For this review, take the finished solid that the model builds, in its own axes (mm). A direction names the side the tool comes from. Coordinates: 2 decimals unless noted, no trailing zeros. Write each loop counter-clockwise with the first axis right and the second up, starting at its lowest first coordinate (ties: lowest second). Pieces come first, ordered by that corner, then holes.
```python
from build123d import *

# Parameters (mm, degrees)
ESBO_O1_W                = 74
ESBO_O1_H                = 20
RESSALTO_EXTRUS_O1_DEPTH = 11
ESBO_O4_W                = 72
ESBO_O4_H                = 9.1
ESBO_O5_W                = 3
ESBO_O5_H                = 3
CORTE_EXTRUS_O2_DEPTH    = 2.5
CORTE_EXTRUS_O3_DEPTH    = 40.874804075
FILETE1_R                = 1
FILETE2_R                = 1
FILETE3_R                = 1
FILETE4_R                = 1
ESBO_O8_W                = 3.2
ESBO_O8_H                = 2
CORTE_EXTRUS_O5_DEPTH    = 44.474130264
FILETE5_R                = 0.5
FILETE6_R                = 0.5
FILETE7_R                = 0.5
FILETE8_R                = 0.5
FILETE5_OF_ESPELHAR3_R   = 0.5
FILETE6_OF_ESPELHAR3_R   = 0.5
FILETE7_OF_ESPELHAR3_R   = 0.5
FILETE8_OF_ESPELHAR3_R   = 0.5


with BuildPart() as part:
    # Esboço1 → Ressalto-extrusão1 (new body)
    with BuildSketch(Plane(origin=(0, 0, 0), x_dir=(1, 0, 0), z_dir=(0, 1, 0))):
        Rectangle(ESBO_O1_W, ESBO_O1_H)
    extrude(amount=RESSALTO_EXTRUS_O1_DEPTH)

    # Esboço4 → Corte-Revolução2 (revolve, cut)
    with BuildSketch(Plane(origin=(0, 11, 0), x_dir=(1, 0, 0), z_dir=(0, 1, 0))):
        with Locations((0, -4.55)):
            Rectangle(ESBO_O4_W, ESBO_O4_H)
    revolve(axis=Axis((-38.336087416, 11, 0), (1, 0, 0)), mode=Mode.SUBTRACT)

    # Esboço5 → Corte-extrusão2 (cut)
    with BuildSketch(Plane(origin=(-36, 0, 0), x_dir=(0, 0, -1), z_dir=(1, 0, 0))):
        with Locations((0, 8)):
            Rectangle(ESBO_O5_W, ESBO_O5_H)
    corte_extrus_o2 = extrude(amount=-CORTE_EXTRUS_O2_DEPTH, mode=Mode.SUBTRACT)

    # Espelhar1: Corte-extrusão2 across plane
    add(corte_extrus_o2.mirror(Plane(origin=(0, 0, 0), x_dir=(0, 0, 1), z_dir=(1, 0, 0))), mode=Mode.SUBTRACT)

    # Esboço6 → Corte-extrusão3 (cut, through all)
    with BuildSketch(Plane(origin=(0, 0, 0), x_dir=(1, 0, 0), z_dir=(0, 1, 0))):
        with BuildLine():
            Line((-36, 2), (-36, -2))
            ThreePointArc((-36, -2), (-34, 0), (-36, 2))
        make_face()
    corte_extrus_o3 = extrude(amount=CORTE_EXTRUS_O3_DEPTH, mode=Mode.SUBTRACT)

    # Filete1
    filete1_edges = [part.edges().sort_by_distance(p)[0] for p in [
        (37, 5.5, 10),
    ]]
    fillet(filete1_edges, radius=FILETE1_R)

    # Filete2
    filete2_edges = [part.edges().sort_by_distance(p)[0] for p in [
        (37, 5.5, -10),
    ]]
    fillet(filete2_edges, radius=FILETE2_R)

    # Filete3
    filete3_edges = [part.edges().sort_by_distance(p)[0] for p in [
        (-37, 5.5, 10),
    ]]
    fillet(filete3_edges, radius=FILETE3_R)

    # Filete4
    filete4_edges = [part.edges().sort_by_distance(p)[0] for p in [
        (-37, 5.5, -10),
    ]]
    fillet(filete4_edges, radius=FILETE4_R)

    # Espelhar2: Corte-extrusão3 across plane
    add(corte_extrus_o3.mirror(Plane(origin=(0, 0, 0), x_dir=(0, 0, 1), z_dir=(1, 0, 0))), mode=Mode.SUBTRACT)

    # Esboço8 → Corte-extrusão5 (cut, through all)
    with BuildSketch(Plane.XY.offset(10)):
        with Locations((-26.6, 2)):
            Rectangle(ESBO_O8_W, ESBO_O8_H)
    corte_extrus_o5 = extrude(amount=-CORTE_EXTRUS_O5_DEPTH, mode=Mode.SUBTRACT)

    # Filete5
    filete5_edges = [part.edges().sort_by_distance(p)[0] for p in [
        (-28.2, 2, 10),
    ]]
    fillet(filete5_edges, radius=FILETE5_R)

    # Filete6
    filete6_edges = [part.edges().sort_by_distance(p)[0] for p in [
        (-25, 2, 10),
    ]]
    fillet(filete6_edges, radius=FILETE6_R)

    # Filete7
    filete7_edges = [part.edges().sort_by_distance(p)[0] for p in [
        (-25, 2, -10),
    ]]
    fillet(filete7_edges, radius=FILETE7_R)

    # Filete8
    filete8_edges = [part.edges().sort_by_distance(p)[0] for p in [
        (-28.2, 2, -10),
    ]]
    fillet(filete8_edges, radius=FILETE8_R)

    # Espelhar3: Corte-extrusão5 across plane
    add(corte_extrus_o5.mirror(Plane(origin=(0, 0, 0), x_dir=(0, 0, 1), z_dir=(1, 0, 0))), mode=Mode.SUBTRACT)

    # Filete5 of Espelhar3
    filete5_of_espelhar3_edges = [part.edges().sort_by_distance(p)[0] for p in [
        (28.2, 2, 10),
    ]]
    fillet(filete5_of_espelhar3_edges, radius=FILETE5_OF_ESPELHAR3_R)

    # Filete6 of Espelhar3
    filete6_of_espelhar3_edges = [part.edges().sort_by_distance(p)[0] for p in [
        (25, 2, 10),
    ]]
    fillet(filete6_of_espelhar3_edges, radius=FILETE6_OF_ESPELHAR3_R)

    # Filete7 of Espelhar3
    filete7_of_espelhar3_edges = [part.edges().sort_by_distance(p)[0] for p in [
        (25, 2, -10),
    ]]
    fillet(filete7_of_espelhar3_edges, radius=FILETE7_OF_ESPELHAR3_R)

    # Filete8 of Espelhar3
    filete8_of_espelhar3_edges = [part.edges().sort_by_distance(p)[0] for p in [
        (28.2, 2, -10),
    ]]
    fillet(filete8_of_espelhar3_edges, radius=FILETE8_OF_ESPELHAR3_R)


solid = part.part
```
Q1. For probe 1 along X at (y, z) = (1.5, 4.5); probe 2 along X at (y, z) = (8, -8); probe 3 along Z at (x, y) = (31, 8.5), list the stretches that pass through material, from the lowest coordinate up.
Ans:
probe 1: x = -37 to -28.2, -25 to 25, 28.2 to 37
probe 2: x = -37 to -36, 36 to 37
probe 3: z = -10 to -8.75, 8.75 to 10
Q2. Add section C-C (z = -6). State the section outline as (x, y) points.
Ans:
outline: (-37, 0) - (37, 0) - (37, 11) - (36, 11) - (36, 4.16) - (-36, 4.16) - (-36, 11) - (-37, 11) - close; hole (-28.2, 1) - (-25, 1) - (-25, 3) - (-28.2, 3) - close; hole (25, 1) - (28.2, 1) - (28.2, 3) - (25, 3) - close
Q3. Add section B-B (y = 4.5). State the section outline as (x, z) points, then the cut area to 3 significant figures.
Ans:
outline: (-37, -9) arc R1 ccw to (-36, -10) - (36, -10) arc R1 ccw to (37, -9) - (37, 9) arc R1 ccw to (36, 10) - (-36, 10) arc R1 ccw to (-37, 9) - close; hole (-36, -6.37) - (36, -6.37) - (36, 6.37) - (-36, 6.37) - close
area: 562 mm2
Q4. Add section D-D (x = -12). State the section outline as (y, z) points.
Ans:
outline: (0, -10) - (11, -10) - (11, -9.1) arc R9.1 cw to (11, 9.1) - (11, 10) - (0, 10) - close
Q5. Tool access review of faces 1 (the cylindrical face through (34, 1, 0)), 2 (the flat face through (36, 5, 0)), 3 (the flat face through (-25, 1.5, 0.1)), 4 (the flat face through (37, 5, 0)), 5 (the flat face through (-1, 5, 10)): name each direction out of +Z, -Z, +X, -X, +Y, -Y from which nothing blocks a thin tool from reaching the whole face with its end or side.
Ans:
face 1: +Y, -Y
face 2: +Y
face 3: +Z, -Z
face 4: +Z, -Z, +X, +Y, -Y
face 5: +Z, +X, -X, +Y, -Y
Q6. Draft analysis for pull direction Y (two halves, no side actions). For faces 6 (the flat face through (-1, 0, 0)), 7 (the flat face through (27, 3, 7)), 8 (the flat face through (-37, 5, 0)), state which applies: +Y half, -Y half, draft (parallel to the pull), parting line (faces both ways), or undercut.
Ans:
face 6: -Y half
face 7: undercut
face 8: draft
Q7. Add section A-A (z = 0). State the section outline as (x, y) points.
Ans:
outline: (-37, 0) - (-36, 0) - (-36, 6.5) - (-37, 6.5) - close; (-37, 9.5) - (-36, 9.5) - (-36, 11) - (-37, 11) - close; (-34, 0) - (34, 0) - (34, 1.9) - (28.2, 1.9) - (28.2, 1) - (25, 1) - (25, 1.9) - (-25, 1.9) - (-25, 1) - (-28.2, 1) - (-28.2, 1.9) - (-34, 1.9) - close; (36, 0) - (37, 0) - (37, 6.5) - (36, 6.5) - close; (36, 9.5) - (37, 9.5) - (37, 11) - (36, 11) - close
Q8. Clearance check with flat-ended pins moving along their axes: pin 1 Ø5 at (x, z) = (-6, -3) entering from +Y; pin 2 Ø0.8 at (x, y) = (36.5, 7.5) entering from +Z (3 decimals); pin 3 Ø0.5 at (x, y) = (36.5, 7.5) entering from -Z. State where each tip first meets the part, or that it passes through.
Ans:
pin 1: stops at y = 3.75
pin 2: stops at z = 9.995
pin 3: stops at z = -9.97
